from build123d import *

# Parameters (mm, degrees)
SKETCH_1_R        = 5.5
SKETCH_1_R_2      = 2.5
EXTRUDE_1_DEPTH   = 15
HOLE_WIZARD_M31_D = 2.5


with BuildPart() as part:
    # Эскиз1 → Бобышка-Вытянуть1 (new body)
    with BuildSketch(Plane.XY):
        Circle(SKETCH_1_R)
        Circle(SKETCH_1_R_2, mode=Mode.SUBTRACT)
    extrude(amount=EXTRUDE_1_DEPTH)

    # Отверстие обработанное метчиком M31 (through all)
    with Locations(Plane.ZY.offset(5.5)):
        with Locations((12, 0), (3, 0)):
            Hole(HOLE_WIZARD_M31_D / 2)


solid = part.part
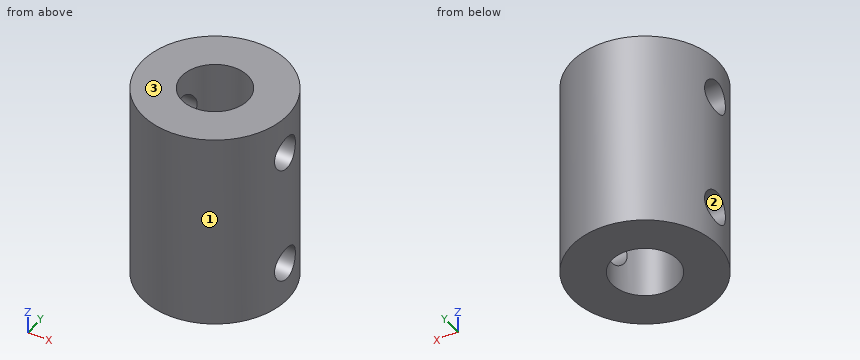
Part model, mm, in its own coordinate system. Face numbers are marked on the shaded views. Give positions to 0.01 mm unless a question says otherwise; leave off trailing zeros. Order: outer loops, then holes, each group sorted by start corner. A loop starts at its lowest first (then second) coordinate and runs counter-clockwise, first axis right, second up. Notation, with made-up numbers: (39, 43.5) -> (93, 43.5) arc R26 ccw to (93, 64.5) -> close; hole circle Ø1 at (-28, 78). An arc over 180 degrees is marked (long way). Use one line per item in the form item = value.
(1) Pull direction Y, two halves, no side cores. Call the marked faces 1, 2 and 3: +Y half, -Y half, draft (parallel to the pull), parting line (faces both ways), or undercut.
Solution:
face_1 = parting line
face_2 = undercut
face_3 = draft
(2) Saw through at D-D (z = 7). Write the cut outline in (x, y).
Solution:
outline = circle Ø11 at (0, 0); hole circle Ø5 at (0, 0)
(3) Drill centre lines: line 1 (Z direction, x = 3.75, y = 0); line 2 (Y direction, x = 0, z = 9.75); line 3 (Z direction, x = -2.5, y = -0.75). Where is each one in solid material? Low to high. Write a range as from..to.
Solution:
line_1 = 0..1.75, 4.25..10.75, 13.25..15
line_2 = -5.5..-2.5, 2.5..5.5
line_3 = 0..2, 4..11, 13..15
(4) Flat gauge pins, fed straight in: P1, Ø1.5, axis at y = -1, z = 6.5, coming from the -X side; P2, Ø2, axis at y = 0, z = 12, coming from the +X side; P3, Ø1, axis at x = -4, z = 2, coming from the +Y side. Where does each tip first touch, or does it go through?
Solution:
P1 = -5.49
P2 = through
P3 = 4.24
(5) Saw through at C-C (z = 12). Write the cut outline in (x, y).
Solution:
outline = (-5.36, -1.25) arc R5.5 ccw to (5.36, -1.25) -> (2.17, -1.25) arc R2.5 cw to (-2.17, -1.25) -> close; (-5.36, 1.25) -> (-2.17, 1.25) arc R2.5 cw to (2.17, 1.25) -> (5.36, 1.25) arc R5.5 ccw to start
(6) Saw through at A-A (x = 0). Write the cut outline in (y, z), then the cut area to 3 significant figures.
Solution:
outline = (-5.5, 0) -> (-2.5, 0) -> (-2.5, 15) -> (-5.5, 15) -> close; (2.5, 0) -> (5.5, 0) -> (5.5, 15) -> (2.5, 15) -> close
area = 90.0 mm²
(7) Saw through at B-B (y = 0). Write the cut outline in (x, z), then the cut area to 3 significant figures.
Solution:
outline = (-5.5, 0) -> (-2.5, 0) -> (-2.5, 1.75) -> (-5.5, 1.75) -> close; (-5.5, 4.25) -> (-2.5, 4.25) -> (-2.5, 10.75) -> (-5.5, 10.75) -> close; (-5.5, 13.25) -> (-2.5, 13.25) -> (-2.5, 15) -> (-5.5, 15) -> close; (2.5, 0) -> (5.5, 0) -> (5.5, 1.75) -> (2.5, 1.75) -> close; (2.5, 4.25) -> (5.5, 4.25) -> (5.5, 10.75) -> (2.5, 10.75) -> close; (2.5, 13.25) -> (5.5, 13.25) -> (5.5, 15) -> (2.5, 15) -> close
area = 60.0 mm²
